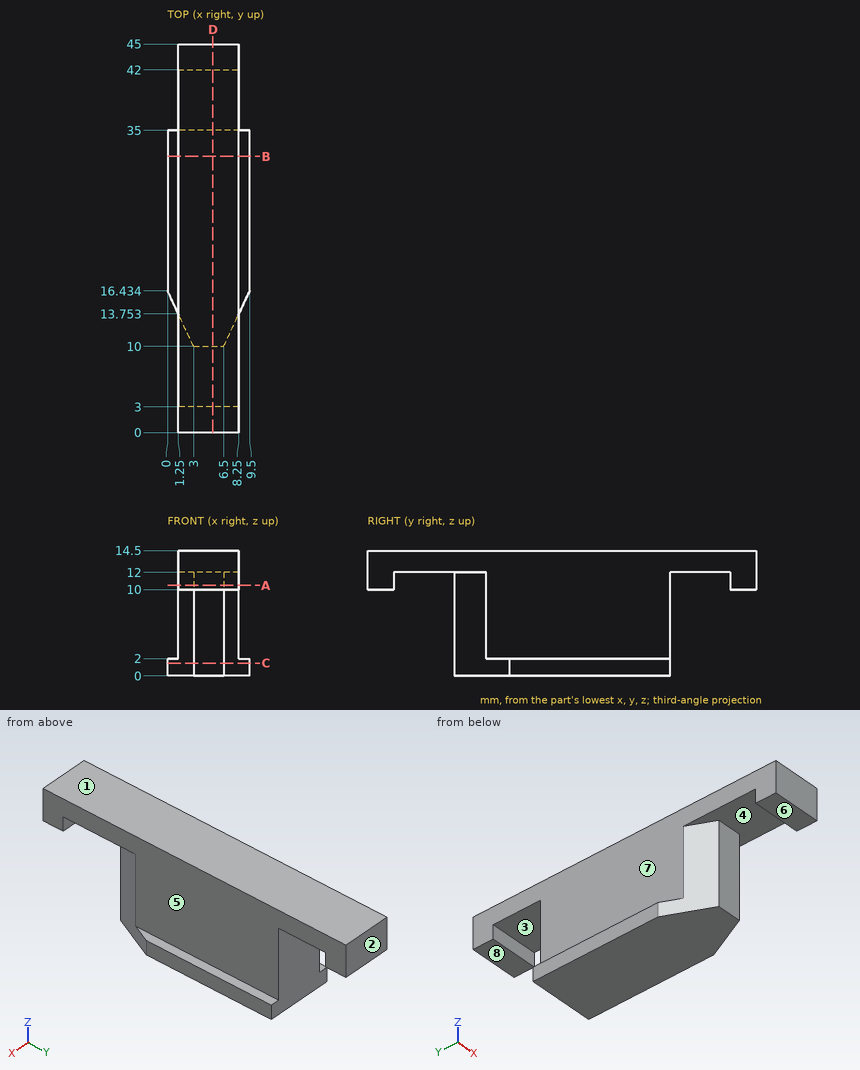
Drawing for the job (mm, zero at the part's lowest x, y, z). A direction names the side the tool comes from. Give positions to 0.01 mm unless a question says otherwise; leave off trailing zeros. Loops run counter-clockwise (first coordinate to the right, second up) from the corner with the lowest first, then second, coordinate; pieces in that order, holes last.
(1) Band-saw the part on D-D (x = 5.25). Write the cut outline in (y, z).
Return value:
outline: (0, 10) - (3, 10) - (3, 12) - (10, 12) - (10, 0) - (35, 0) - (35, 12) - (42, 12) - (42, 10) - (45, 10) - (45, 14.5) - (0, 14.5) - close
(2) Band-saw the part on B-B (y = 32). Write the cut outline in (x, z), and give its area (4 significant figures).
Return value:
outline: (0, 0) - (9.5, 0) - (9.5, 2) - (8.25, 2) - (8.25, 14.5) - (1.25, 14.5) - (1.25, 2) - (0, 2) - close
area: 106.5 mm2
(3) Pin check, flat tips, straight feed: pin 1 (2.5 mm diameter, centred on x = 5.5, y = 1, fed in from -Z); pin 2 (4 mm diameter, centred on y = 20.5, z = 10.5, fed in from -X); pin 3 (6 mm diameter, centred on y = 9.5, z = 5, fed in from +X) (1 decimal). Stop position of each tip, or through.
Return value:
pin 1: stops at z = 10
pin 2: stops at x = 1.25
pin 3: stops at x = 7.7
(4) Band-saw the part on C-C (z = 1.5). Write the cut outline in (x, y).
Return value:
outline: (0, 16.43) - (3, 10) - (6.5, 10) - (9.5, 16.43) - (9.5, 35) - (0, 35) - close
(5) Pull direction Y, two halves, no side cores. Call the marked faces 1, 2, 3 and 4: pulls with the +Y half, pulls with the -Y half, needs draft (parallel to the pull), parting line crosses it, or undercut.
Return value:
face 1: needs draft
face 2: pulls with the +Y half
face 3: undercut
face 4: undercut
(6) Band-saw the part on A-A (z = 10.5). Write the cut outline in (x, y).
Return value:
outline: (1.25, 0) - (8.25, 0) - (8.25, 3) - (1.25, 3) - close; (1.25, 13.75) - (3, 10) - (6.5, 10) - (8.25, 13.75) - (8.25, 35) - (1.25, 35) - close; (1.25, 42) - (8.25, 42) - (8.25, 45) - (1.25, 45) - close
(7) 3-axis set-ups, long thin cutter, end or side, ignore diameter. For the marked faces 5, 6, 7 and 8: which of +Z, -Z, +X, -X, +Y, -Y reach the whole face in a straight line?
Return value:
face 5: +Z, +X, +Y, -Y
face 6: -Z, +X, -X, -Y
face 7: +Z, -X, +Y, -Y
face 8: -Z, +X, -X, +Y
(8) Drill centre lines: line 1 along Y through (x, z) = (4.75, 11.25); line 2 along Y through (x, z) = (2, 10.75) (1 decimal); line 3 along X through (y, z) = (25, 10). Where is each one in solid material? Low to high.
Return value:
line 1: y = 0 to 3, 10 to 35, 42 to 45
line 2: y = 0 to 3, 12.1 to 35, 42 to 45
line 3: x = 1.25 to 8.25
